The drawing under review shows one solid part. Ordinate dimensions are in mm from its lowest x, y, z. A direction names the side the tool comes from. Give positions to 0.01 mm unless a question says otherwise; leave off trailing zeros. Write each loop counter-clockwise with the first axis right and the second up, starting at its lowest first coordinate (ties: lowest second). Pieces come first, ordered by that corner, then holes.
Q1. We need section D-D (x = 17.25). Write out the cut boundary in (y, z).
Q2. We need section A-A (x = 10). Write out the cut boundary in (y, z).
Q3. Mouldability with a two-part tool opening along Y and no side actions: class the marked faces 6, 7 and 8 as released by +Y, released by -Y, zero draft, split by the parting line, or undercut.
Q4. We need section B-B (y = 20). Write out the cut boundary in (x, z).
Q5. Insertion check: P1, Ø4.5, axis at x = 10, y = 14.5, coming from the +Z side; P2, Ø4, axis at x = 18, z = 4.5, coming from the -Y side; P3, Ø1, axis at y = 8.5, z = 12.5, coming from the +X side; P4, Ø10, axis at x = 14.5, y = 31, coming from the +Z side. Each pin has a flat end and moves straight along its axis. Give the tip position at first contact, or say it passes through.
Q6. We need section C-C (z = 22.25). Write out the cut boundary in (x, y), then the cut area to 4 significant figures.
Q7. Machinability: for the marked faces 1, 2, 3, 4 and 5, which of the approach directions +Z, -Z, +X, -X, +Y, -Y give a long, thin tool a straight path to every point of the face, cutting with its end or side? Answer none if there is none.
Q8. For line 1 (Y direction, x = 10, z = 4.35); line 2 (X direction, y = 20, z = 0.8); line 3 (Y direction, x = 10, z = 1.7), list the stretches that pass through material, from the lowest coordinate up.
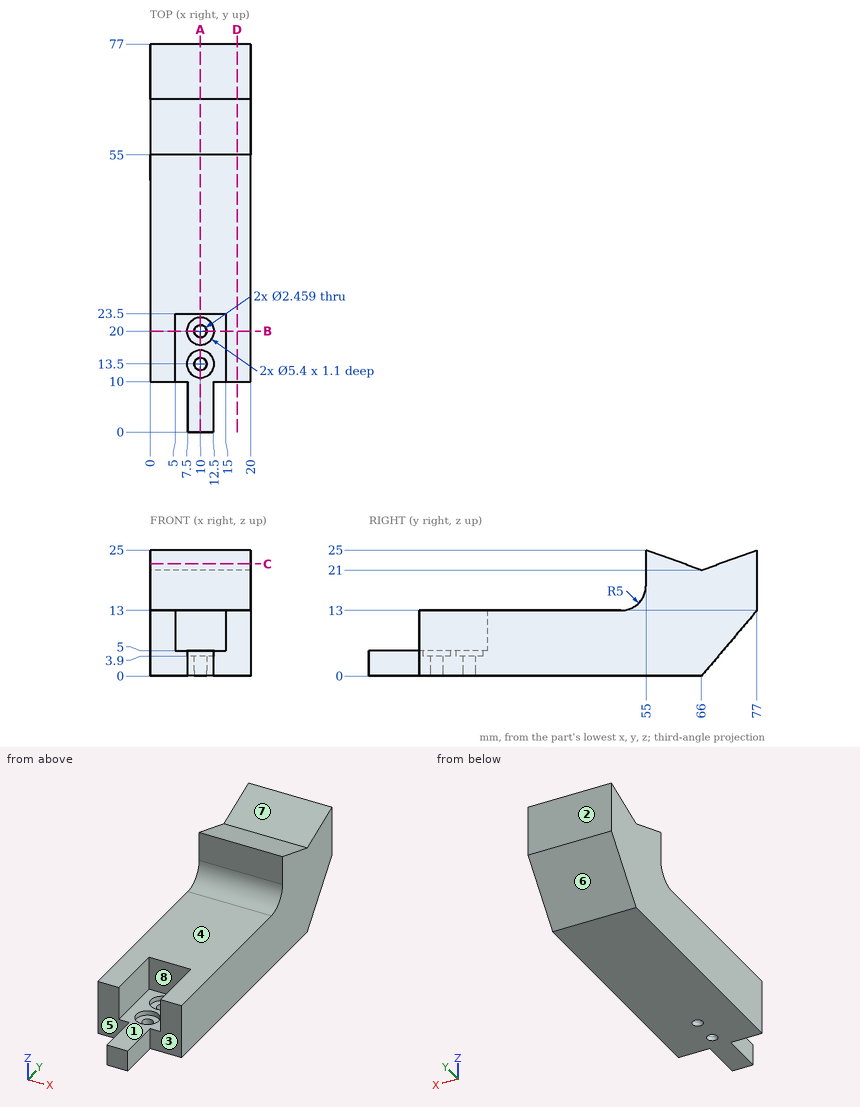
Computed:
1. outline: (10, 0) - (66, 0) - (77, 13) - (77, 25) - (66, 21) - (55, 25) - (55, 18) arc R5 cw to (50, 13) - (10, 13) - close
2. outline: (0, 0) - (12.27, 0) - (12.27, 3.9) - (10.8, 3.9) - (10.8, 5) - (0, 5) - close; (14.73, 0) - (18.77, 0) - (18.77, 3.9) - (17.3, 3.9) - (17.3, 5) - (16.2, 5) - (16.2, 3.9) - (14.73, 3.9) - close; (21.23, 0) - (66, 0) - (77, 13) - (77, 25) - (66, 21) - (55, 25) - (55, 18) arc R5 cw to (50, 13) - (23.5, 13) - (23.5, 5) - (22.7, 5) - (22.7, 3.9) - (21.23, 3.9) - close
3. face 6: released by +Y
3. face 7: undercut
3. face 8: released by -Y
4. outline: (0, 0) - (8.77, 0) - (8.77, 3.9) - (7.3, 3.9) - (7.3, 5) - (5, 5) - (5, 13) - (0, 13) - close; (11.23, 0) - (20, 0) - (20, 13) - (15, 13) - (15, 5) - (12.7, 5) - (12.7, 3.9) - (11.23, 3.9) - close
5. P1: stops at z = 5
5. P2: stops at y = 10
5. P3: passes through
5. P4: stops at z = 13
6. outline: (0, 55) - (20, 55) - (20, 62.56) - (0, 62.56) - close; (0, 69.44) - (20, 69.44) - (20, 77) - (0, 77) - close
6. area: 302.5 mm2
7. face 1: +Z, -Y
7. face 2: +Z, -Z, +X, -X, +Y
7. face 3: +Z, -Z, +X, -Y
7. face 4: +Z, +X, -X, -Y
7. face 5: +Z, -Z, -X, -Y
8. line 1: y = 0 to 10.8, 16.2 to 17.3, 22.7 to 69.68
8. line 2: x = 0 to 8.77, 11.23 to 20
8. line 3: y = 0 to 12.27, 14.73 to 18.77, 21.23 to 67.44
